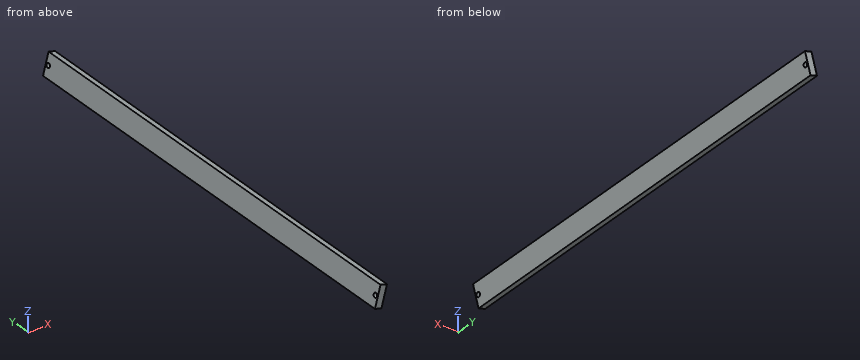
from build123d import *

# Parameters (mm, degrees)
BOSS_EXTRUDE1_DEPTH = 431.8
SKETCH2_R           = 2.0955
CUT_EXTRUDE1_DEPTH  = 433.042370256
SKETCH3_R           = 2.0955
CUT_EXTRUDE2_DEPTH  = 433.042370256


with BuildPart() as part:
    # Sketch1 → Boss-Extrude1 (new body)
    with BuildSketch(Plane(origin=(0, 0, 0), x_dir=(1, 0, 0), z_dir=(0, 1, 0))):
        Polygon((39.444022474, 0), (45.577651471, 1.643500936), (40.293154487, 21.365512173), (34.15952549, 19.722011237), align=None)
    extrude(amount=BOSS_EXTRUDE1_DEPTH)

    # Sketch2 → Cut-Extrude1 (cut, through all)
    with BuildSketch(Plane(origin=(36.801773982, 0, -9.861005618), x_dir=(0.25881904510252096, 0, 0.9659258262890683), z_dir=(-0.9659258262890683, 0, 0.25881904510252096))):
        with Locations((0, 428.625)):
            Circle(SKETCH2_R)
    extrude(amount=-CUT_EXTRUDE1_DEPTH, mode=Mode.SUBTRACT)

    # Sketch3 → Cut-Extrude2 (cut, through all)
    with BuildSketch(Plane(origin=(36.801773982, 0, -9.861005618), x_dir=(0.25881904510252096, 0, 0.9659258262890683), z_dir=(-0.9659258262890683, 0, 0.25881904510252096))):
        with Locations((0, 3.175)):
            Circle(SKETCH3_R)
    extrude(amount=-CUT_EXTRUDE2_DEPTH, mode=Mode.SUBTRACT)


solid = part.part
The listing builds one solid part. Answer for the finished solid, in the listing's coordinates (mm). Give positions to 0.01 mm unless a question says otherwise; leave off trailing zeros. Order: outer loops, then holes, each group sorted by start corner. A loop starts at its lowest first (then second) coordinate and runs counter-clockwise, first axis right, second up. Notation, with made-up numbers: (2, 88.5) -> (57, 88.5) arc R24 cw to (57, 121.5) -> close; hole circle Ø8 at (-14, 72). An arc over 180 degrees is marked (long way). Put each result on its own line as item: value.
Item 1: Straight lines are drawn through the part: line 1 (Y direction, x = 38.5, z = -10); line 2 (X direction, y = 55, z = -5.5); line 3 (X direction, y = 336, z = -10). For each, find the intervals that lie inside material, in ascending order.
Established:
line 1: y = 0 to 1.1, 5.25 to 426.55, 430.7 to 431.8
line 2: x = 37.97 to 44.54
line 3: x = 36.76 to 43.34
Item 2: Given P1, Ø12, axis at y = 118, z = -10, coming from the +X side; P2, Ø10, axis at y = 217, z = -19, coming from the -X side; P3, Ø2, axis at y = 151.5, z = -8.5, coming from the +X side; P4, Ø1, axis at x = 43, y = 362.5, coming from the +Z side, each flat-ended and moving along its own axis, determine where each tip first touches the part or whether it passes through.
Established:
P1: stops at x = 44.95
P2: stops at x = 34.16
P3: stops at x = 44.01
P4: stops at z = -0.82
Item 3: A cutting plane is placed at A-A on y = 324. Give the vertices of the cut face in (x, z), plus the area to 3 significant figures.
Established:
outline: (34.16, -19.72) -> (40.29, -21.37) -> (45.58, -1.64) -> (39.44, 0) -> close
area: 130 mm^2
